Here's how the part is built. I have some questions about the finished solid (model axes, mm). Round coordinates to 2 decimals unless told otherwise and drop trailing zeros. Loops run counter-clockwise (first coordinate to the right, second up) from the corner with the lowest first, then second, coordinate; pieces in that order, holes last. Notation, with made-up numbers: M 69,3.5 L 103,3.5 A17 ccw 103,17.5 Z; hole C -35,81 d2. An arc over 180 degrees is marked long. Answer as a JSON object with one key per item and string values.
from build123d import *

# Parameters (mm, degrees)
SKETCH1_R           = 146.05
SKETCH1_R_2         = 3.175
SKETCH1_R_3         = 2.8575
SKETCH1_R_4         = 15.875
SKETCH1_R_5         = 12.7
BOSS_EXTRUDE1_DEPTH = 6.35


with BuildPart() as part:
    # Sketch1 → Boss-Extrude1 (new body)
    with BuildSketch(Plane.XY):
        Circle(SKETCH1_R)
        with Locations((0, 136.525)):
            Circle(SKETCH1_R_2, mode=Mode.SUBTRACT)
        with Locations((136.525, 0)):
            Circle(SKETCH1_R_2, mode=Mode.SUBTRACT)
        with Locations((0, -136.525)):
            Circle(SKETCH1_R_2, mode=Mode.SUBTRACT)
        with Locations((-136.525, 0)):
            Circle(SKETCH1_R_2, mode=Mode.SUBTRACT)
        with Locations((-30.226, 46.482)):
            Circle(SKETCH1_R_3, mode=Mode.SUBTRACT)
        with Locations(Location((30.226, 46.482, 0), (0, 0, 180))):
            Circle(SKETCH1_R_3, mode=Mode.SUBTRACT)
        with Locations((30.226, -17.018)):
            Circle(SKETCH1_R_3, mode=Mode.SUBTRACT)
        with Locations(Location((-30.226, -17.018, 0), (0, 0, 180))):
            Circle(SKETCH1_R_3, mode=Mode.SUBTRACT)
        Circle(SKETCH1_R_4, mode=Mode.SUBTRACT)
        with Locations((0, 60.325)):
            Circle(SKETCH1_R_5, mode=Mode.SUBTRACT)
        with Locations((60.325, 0)):
            Circle(SKETCH1_R_5, mode=Mode.SUBTRACT)
        with Locations((0, -60.325)):
            Circle(SKETCH1_R_5, mode=Mode.SUBTRACT)
        with Locations((-60.325, 0)):
            Circle(SKETCH1_R_5, mode=Mode.SUBTRACT)
    extrude(amount=BOSS_EXTRUDE1_DEPTH)


solid = part.part
Item 1: I want a section at C-C, the plane y = 116.5. Please give me the cut outline in (x, z).
Resolved:
{"outline": "M -88.08,0 L 88.08,0 L 88.08,6.35 L -88.08,6.35 Z"}
Item 2: Please list where these lines run through material, in increasing order: probe 1 along Y at (x, z) = (0, 2) (3 decimals); probe 2 along X at (y, z) = (-5, 1.5); probe 3 along Y at (x, z) = (-6.5, 5). Write a range as from..to.
Resolved:
{"probe 1": "-146.05..-139.7, -133.35..-73.025, -47.625..-15.875, 15.875..47.625, 73.025..133.35, 139.7..146.05", "probe 2": "-145.96..-72, -48.65..-15.07, 15.07..48.65, 72..145.96", "probe 3": "-145.91..-71.24, -49.41..-14.48, 14.48..49.41, 71.24..145.91"}
Item 3: I want a section at D-D, the plane y = -80. Please give me the cut outline in (x, z), then the cut area to 3 significant figures.
Resolved:
{"outline": "M -122.19,0 L 122.19,0 L 122.19,6.35 L -122.19,6.35 Z", "area": "1,550 mm²"}
Item 4: I want a section at A-A, the plane y = -8. Please give me the cut outline in (x, z), then the cut area to 3 significant figures.
Resolved:
{"outline": "M -145.83,0 L -70.19,0 L -70.19,6.35 L -145.83,6.35 Z; M -50.46,0 L -13.71,0 L -13.71,6.35 L -50.46,6.35 Z; M 13.71,0 L 50.46,0 L 50.46,6.35 L 13.71,6.35 Z; M 70.19,0 L 145.83,0 L 145.83,6.35 L 70.19,6.35 Z", "area": "1,430 mm²"}
Item 5: If we mould it in two halves opening along X, with no side actions, what happens to faces 1 (the face through (-133.592, -1.216, 3.131)), 2 (the face through (139.306, 43.869, 3.131)), 3 (the face through (-2, -30, 0))? For each: pulls with the +X half, pulls with the -X half, needs draft (parallel to the pull), parting line crosses it, or undercut.
Resolved:
{"face 1": "undercut", "face 2": "parting line crosses it", "face 3": "needs draft"}
Item 6: I want a section at B-B, the plane z = 1.25. State how many separate pieces and enclosed holes the cut face has, then the cut area to 3 significant figures.
Resolved:
{"separate pieces": "1", "enclosed holes": "13", "area": "64,000 mm²"}
Item 7: I'm going to push flat-ended pins straight in: pin 1 Ø4 at (x, y) = (0, 136.525) entering from +Z; pin 2 Ø9 at (x, y) = (-30.226, -17.018) entering from -Z. Where does each tip first touch, or does it pass through?
Resolved:
{"pin 1": "through", "pin 2": "z = 0"}
